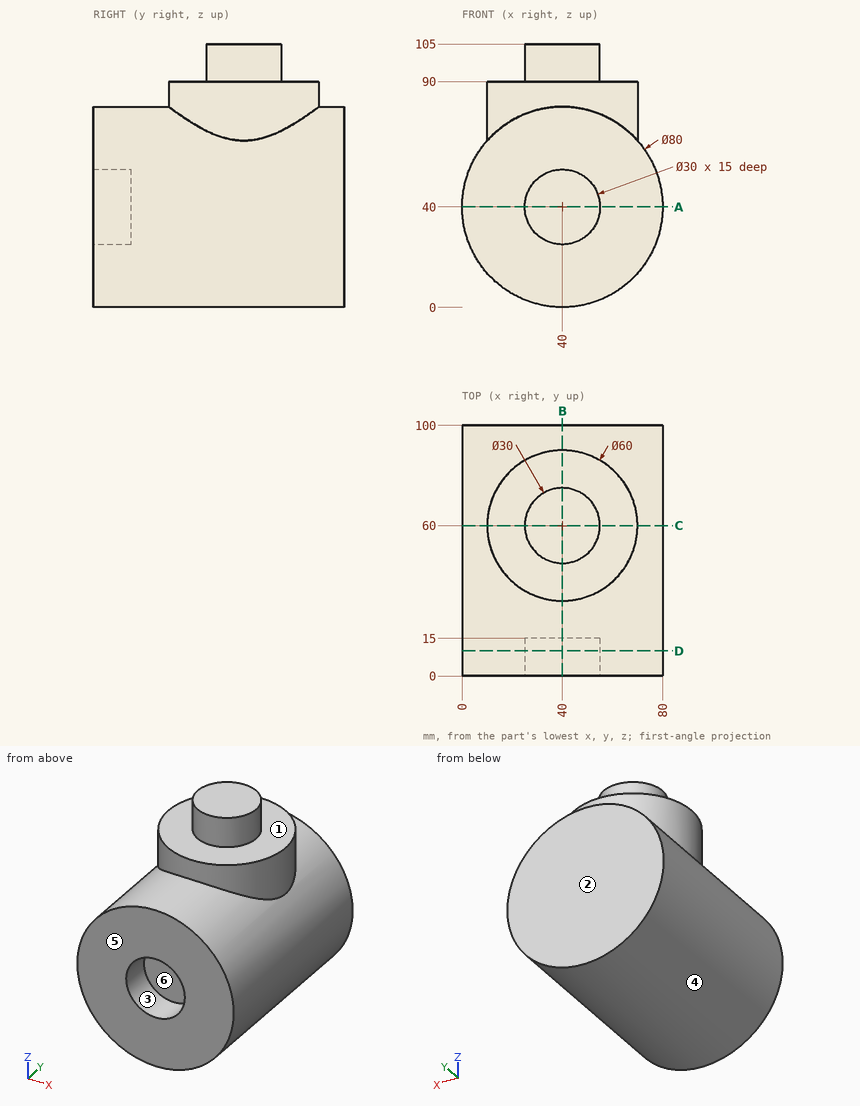
Source: three-view drawing plus pictorial views. Frame: mm from the lowest corner of the part. A direction names the side the tool comes from. Round coordinates to 2 decimals unless told otherwise and drop trailing zeros. Loops run counter-clockwise (first coordinate to the right, second up) from the corner with the lowest first, then second, coordinate; pieces in that order, holes last. Notation, with made-up numbers: (70, 75) -> (90, 75) arc R10 ccw to (90, 81) -> close; hole circle Ø2 at (17, 68). An arc over 180 degrees is marked (long way). Use one line per item in the form item = value.
Item 1: Cut plane A-A on z = 40. Output: boundary loops of the cut face in (x, y).
Evaluation:
outline = (0, 0) -> (25, 0) -> (25, 15) -> (55, 15) -> (55, 0) -> (80, 0) -> (80, 100) -> (0, 100) -> close
Item 2: Cut plane D-D on y = 10. Output: boundary loops of the cut face in (x, z).
Evaluation:
outline = circle Ø80 at (40, 40); hole circle Ø30 at (40, 40)
Item 3: Draft query along Z for the marked faces 4, 5 and 6. Return one class per face: released by +Z, released by -Z, zero draft, split by the parting line, or undercut.
Evaluation:
face_4 = split by the parting line
face_5 = zero draft
face_6 = undercut
Item 4: Cut plane C-C on y = 60. Output: boundary loops of the cut face in (x, z).
Evaluation:
outline = (10, 66.46) arc R40 ccw (long way) to (70, 66.46) -> (70, 90) -> (55, 90) -> (55, 105) -> (25, 105) -> (25, 90) -> (10, 90) -> close
Item 5: Contact query for flat-ended pins moving along their axis: pin 1 Ø12 at (y, z) = (23.5, 14) entering from +X; pin 2 Ø5 at (x, y) = (70, 15) entering from -Z; pin 3 Ø12 at (x, y) = (28, 19) entering from -Z. Output: stop coordinate, or through.
Evaluation:
pin_1 = 74.64
pin_2 = 10.95
pin_3 = 0.45
Item 6: Access query for the marked faces 1, 2 and 3. Directions: +Z, -Z, +X, -X, +Y, -Y. A direction counts if a zero-diameter tool reaches every point of the face in a straight line with its end or side. Return the directions, or none.
Evaluation:
face_1 = +Z
face_2 = +Z, -Z, +X, -X, +Y
face_3 = -Y
Item 7: Material intervals for probe 1 along X at (y, z) = (10.5, 40); probe 2 along Y at (x, z) = (28.5, 37); probe 3 along X at (y, z) = (8, 26.5), sorted ascending.
Evaluation:
probe_1 = 0 to 25, 55 to 80
probe_2 = 15 to 100
probe_3 = 2.35 to 33.46, 46.54 to 77.65
Item 8: Cut plane B-B on x = 40. Output: boundary loops of the cut face in (y, z), then the cut area to 3 significant figures.
Evaluation:
outline = (0, 0) -> (100, 0) -> (100, 80) -> (90, 80) -> (90, 90) -> (75, 90) -> (75, 105) -> (45, 105) -> (45, 90) -> (30, 90) -> (30, 80) -> (0, 80) -> (0, 55) -> (15, 55) -> (15, 25) -> (0, 25) -> close
area = 8,600 mm2
